from build123d import *

# Parameters (mm, degrees)
F1_DEPTH = 50.8
F2_R     = 5.08
F3_SIZE  = 5.08


with BuildPart() as f1:
    # F0 (on Top) → F1 (new body)
    with BuildSketch(Plane.XY):
        with BuildLine():
            Line((25.4, 0), (0, 0))
            Line((0, 0), (0, -50.8))
            Line((0, -50.8), (25.4, -50.8))
            Line((25.4, -50.8), (25.4, -30.870903))
            ThreePointArc((25.4, -30.870903), (17.7038, -23.174703), (25.4, -15.478503))
            Line((25.4, -15.478503), (25.4, 0))
        make_face()
        with BuildLine():
            Line((46.007535, -14.848889), (25.4, 0))
            Line((25.4, 0), (25.4, -15.478503))
            ThreePointArc((25.4, -15.478503), (30.842035, -17.732668), (33.0962, -23.174703))
            ThreePointArc((33.0962, -23.174703), (30.842035, -28.616738), (25.4, -30.870903))
            Line((25.4, -30.870903), (25.4, -50.8))
            Line((25.4, -50.8), (46.007535, -14.848889))
        make_face()
    extrude(amount=F1_DEPTH)

    # F2
    f2_edges = [f1.edges().sort_by_distance(p)[0] for p in [
        (25.4, -50.8, 25.4),
    ]]
    fillet(f2_edges, radius=F2_R)

    # F3
    f3_edges = [f1.edges().sort_by_distance(p)[0] for p in [
        (46.007535, -14.848889, 25.4),
    ]]
    chamfer(f3_edges, length=F3_SIZE)


solid = f1.part
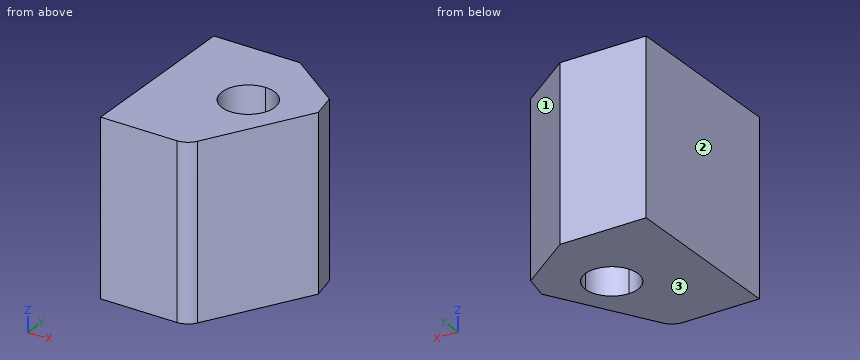
Could you check a few things on this model? Use its own coordinates, in mm. Face numbers are marked on the shaded views. Round coordinates to 2 decimals unless told otherwise and drop trailing zeros. Order: outer loops, then holes, each group sorted by start corner. A loop starts at its lowest first (then second) coordinate and runs counter-clockwise, first axis right, second up.
Q1. Imagine slicing it at D-D, the plane y = -40. List the corners of the cut face in (x, z) for me, then the cut area to 3 significant figures.
Geometry says:
outline: (0, 0) - (31.59, 0) - (31.59, 50.8) - (0, 50.8) - close
area: 1,600 mm2
Q2. Imagine slicing it at C-C, the plane x = 28.5. List the corners of the cut face in (y, z) for me.
Geometry says:
outline: (-45.39, 0) - (-30.22, 0) - (-30.22, 50.8) - (-45.39, 50.8) - close; (-16.13, 0) - (-2.23, 0) - (-2.23, 50.8) - (-16.13, 50.8) - close
Q3. Imagine slicing it at A-A, the plane y = -27. List the corners of the cut face in (x, z) for me.
Geometry says:
outline: (0, 0) - (18.72, 0) - (18.72, 50.8) - (0, 50.8) - close; (32.08, 0) - (39.04, 0) - (39.04, 50.8) - (32.08, 50.8) - close
Q4. I'm going to push flat-ended pins straight in: P1, Ø8, axis at x = 13.5, z = 17, coming from the +Y side; P2, Ø4, axis at x = 38.5, z = 22, coming from the +Y side; P3, Ø4, axis at y = -12.5, z = 30, coming from the +X side; P4, Ø6, axis at y = -37.5, z = 30, coming from the +X side. Where does each tip first touch, or does it pass through?
Geometry says:
P1: stops at y = 0
P2: stops at y = -8
P3: stops at x = 42.45
P4: stops at x = 34.74
Q5. Please list where these lines run through material, in increasing order: probe 1 along Y at (x, z) = (30.5, 19.5); probe 2 along X at (y, z) = (-28, 18); probe 3 along Y at (x, z) = (21.5, 35).
Geometry says:
probe 1: y = -41.9 to -28.94, -17.41 to -3.67
probe 2: x = 0 to 19.4, 31.4 to 38.47
probe 3: y = -50.8 to -29.81, -16.54 to 0
Q6. Thinking about a two-plate mould opening in X: for the marked faces 1, 2 and 3, which applies, released by +X, released by -X, zero draft, split by the parting line, or undercut?
Geometry says:
face 1: released by +X
face 2: released by -X
face 3: zero draft
Q7. Imagine slicing it at B-B, the plane z = 10. List the corners of the cut face in (x, y) for me.
Geometry says:
outline: (0, -50.8) - (22.46, -50.8) arc R5.08 ccw to (26.86, -48.25) - (43.48, -19.26) - (41.89, -11.88) - (25.4, 0) - (0, 0) - close; hole (25.4, -15.48) arc R7.7 ccw (long way) to (33.1, -23.17) arc R7.7 ccw to start
